from build123d import *

# Parameters (mm, degrees)
SKETCH2_R           = 2.5
BOSS_EXTRUDE1_DEPTH = 5
FILLET1_R           = 2


with BuildPart() as part:
    # Sketch2 → Boss-Extrude1 (new, symmetric)
    with BuildSketch(Plane.XY):
        with BuildLine():
            Line((-1, 15), (1, 15))
            ThreePointArc((1, 15), (3.237065366, 9.584445672), (4, 3.774917218))
            ThreePointArc((4, 3.774917218), (5.050348735, -2.178067412), (0, -5.5))
            ThreePointArc((0, -5.5), (-50.58302006, -1.652596692), (-100.002221288, 9.801091818))
            ThreePointArc((-100.002221288, 9.801091818), (-101.650418114, 12.901978174), (-98.572266253, 14.592253326))
            ThreePointArc((-98.572266253, 14.592253326), (-52.235024066, 5.027100207), (-5, 2.291287847))
            ThreePointArc((-5, 2.291287847), (-4.560733387, 3.074038219), (-4, 3.774917218))
            ThreePointArc((-4, 3.774917218), (-3.237065366, 9.584445672), (-1, 15))
        make_face()
        Circle(SKETCH2_R, mode=Mode.SUBTRACT)
    extrude(amount=BOSS_EXTRUDE1_DEPTH, both=True)

    # Fillet1
    # the kernel refuses this fillet: 2 mm, written as the material it takes off along each edge
    with BuildSketch(Plane(origin=(1, 15, 8.124355519), x_dir=(0.4746222349820919, -0.8801896011999936, 0), z_dir=(0, 0, -1))) as fillet1_piece_1:
        with BuildLine():
            CenterArc((1.194199131, 1.999228593), FILLET1_R, 208.334756637, 63.256639898)
            Line((-0.566180071, 1.049984123), (0, 0))
            ThreePointArc((0, 0), (0.624871104, -0.00867849), (1.249742207, 0))
        make_face()
    extrude(amount=16.248711037, mode=Mode.SUBTRACT)
    with BuildSketch(Plane(origin=(-1, 15, 8.124355519), x_dir=(1, 0, 0), z_dir=(0, 0, -1))) as fillet1_piece_2:
        with BuildLine():
            CenterArc((1.192906757, 2), FILLET1_R, 206.743360102, 63.256639898)
            ThreePointArc((-0.59315544, 1.100010095), (-0.304216436, 0.545886044), (0, 0))
            Line((0, 0), (1.192906757, 0))
        make_face()
    extrude(amount=16.248711037, mode=Mode.SUBTRACT)


solid = part.part
Part model, mm, in its own coordinate system. A direction names the side the tool comes from. Give positions to 0.01 mm unless a question says otherwise; leave off trailing zeros. Loops run counter-clockwise (first coordinate to the right, second up) from the corner with the lowest first, then second, coordinate; pieces in that order, holes last. Notation, with made-up numbers: M 66.5,-40 L 95.5,-40 A23 cw 95.5,-23 Z; hole C 60.5,38.25 d4. An arc over 180 degrees is marked long. Put each result on its own line as item: value. Start each with the question number.
1) Saw through at C-C (y = 7). List the corners of the cut face in (x, z), then the cut area to 3 significant figures.
2) Saw through at A-A (z = 1.5). List the corners of the cut face in (x, y).
3) Saw through at B-B (y = 13). List the corners of the cut face in (x, z).
4) Probe probe 1 along Y at (x, z) = (-13, 4.25); probe 2 along Y at (x, z) = (-48, -2.75). List the from-to ranges inside material, lowest first.
5) Saw through at D-D (x = -54.5). List the corners of the cut face in (y, z), then the cut area to 3 significant figures.
6) Flat gauge pins, fed straight in: pin 1 (5 mm diameter, centred on y = 3.5, z = 2, fed in from +X); pin 2 (3 mm diameter, centred on x = -30, z = 0, fed in from +Y); pin 3 (6 mm diameter, centred on y = 7, z = -3.5, fed in from +X). Where does each tip first touch, or does it go through?
7) Pull direction Y, two halves, no side cores. Call faces 3 (the cylindrical face through (-52.892, 5.114, 0.07)), 4 (the cylindrical face through (-101.665, 12.85, 0.07)), 5 (the flat face through (-40, 3, 5)), 6 (the cylindrical face through (-0.54, -2.44, -0.07)): +Y half, -Y half, draft (parallel to the pull), parting line (faces both ways), or undercut.
8) 3-axis set-ups, long thin cutter, end or side, ignore diameter. For faces 1 (the cylindrical face through (5.085, -2.096, 0.07)), 2 (the cylindrical face through (-3.407, 8.907, 0.07)): which of +Z, -Z, +X, -X, +Y, -Y reach the whole face in a straight line?
Numbers:
1. outline: M -90.58,-5 L -65.21,-5 L -65.21,5 L -90.58,5 Z; M -3.77,-5 L 3.77,-5 L 3.77,5 L -3.77,5 Z
1. area: 329 mm^2
2. outline: M -100,9.8 A334.44 ccw 0,-5.5 A5.5 ccw 4,3.77 A22.5 ccw 1.59,13.9 A2 ccw 0,14.99 A2 ccw -1.59,13.9 A22.5 ccw -4,3.77 A5.5 ccw -5,2.29 A325 cw -98.57,14.59 A2.5 ccw Z; hole C 0,0 d5
3. outline: M -101.62,-5 L -92.75,-5 L -92.75,5 L -101.62,5 Z; M -2.02,-5 L 2.02,-5 L 2.02,5 L -2.02,5 Z
4. probe 1: -5.25 to 2.27
4. probe 2: -2.04 to 4.5
5. outline: M -1.03,-5 L 5.33,-5 L 5.33,5 L -1.03,5 Z
5. area: 63.6 mm^2
6. pin 1: x = 5.41
6. pin 2: y = 2.97
6. pin 3: x = 4
7. face 3: +Y half
7. face 4: parting line
7. face 5: draft
7. face 6: undercut
8. face 1: +Z, -Z, +X
8. face 2: +Z, -Z, +Y
